Source: CAD feature listing. Evaluate the final solid. Frame: model axes, mm. A direction names the side the tool comes from. Give positions to 0.01 mm unless a question says otherwise; leave off trailing zeros. Loops run counter-clockwise (first coordinate to the right, second up) from the corner with the lowest first, then second, coordinate; pieces in that order, holes last. Notation, with made-up numbers: M -13.5,31.5 L -9.5,31.5 A19 cw -9.5,49.5 Z; hole C -38.5,30.25 d9. An arc over 180 degrees is marked long. Put each result on its own line as item: value. Start each with the question number.
```python
from build123d import *

# Parameters (mm, degrees)
EXTRUDE_1_DEPTH     = 28
SKETCH_2_R          = 11
EXTRUDE_2_DEPTH     = 2
SKETCH_3_R          = 2.5
EXTRUDE_3_DEPTH     = 13
SKETCH_4_R          = 1.3
CUT_EXTRUDE_1_DEPTH = 5


with BuildPart() as part:
    # 草图1 → 凸台-拉伸1 (new body)
    with BuildSketch(Plane(origin=(0, 0, 0), x_dir=(1, 0, 0), z_dir=(0, 1, 0))):
        with BuildLine():
            Line((-11.5, 14), (11.5, 14))
            ThreePointArc((11.5, 14), (13.267766953, 13.267766953), (14, 11.5))
            Line((14, 11.5), (14, -11.5))
            ThreePointArc((14, -11.5), (13.267766953, -13.267766953), (11.5, -14))
            Line((11.5, -14), (-11.5, -14))
            ThreePointArc((-11.5, -14), (-13.267766953, -13.267766953), (-14, -11.5))
            Line((-14, -11.5), (-14, 11.5))
            ThreePointArc((-14, 11.5), (-13.267766953, 13.267766953), (-11.5, 14))
        make_face()
    extrude(amount=EXTRUDE_1_DEPTH)

    # 草图2 → 凸台-拉伸2 (add)
    with BuildSketch(Plane(origin=(0, 28, 0), x_dir=(-1, 0, 0), z_dir=(0, 1, 0))):
        with Locations(Location((0, 0, 0), (0, 0, 90))):
            Circle(SKETCH_2_R)
    extrude(amount=EXTRUDE_2_DEPTH)

    # 草图3 → 凸台-拉伸3 (add)
    with BuildSketch(Plane(origin=(0, 30, 0), x_dir=(-1, 0, 0), z_dir=(0, 1, 0))):
        with Locations(Location((0, 0, 0), (0, 0, 270))):
            Circle(SKETCH_3_R)
    extrude(amount=EXTRUDE_3_DEPTH)

    # 草图4 → 切除-拉伸1 (cut)
    with BuildSketch(Plane(origin=(0, 28, 0), x_dir=(-1, 0, 0), z_dir=(0, 1, 0))):
        with Locations(Location((11.5, 11.5, 0), (0, 0, 90))):
            Circle(SKETCH_4_R)
        with Locations(Location((11.5, -11.5, 0), (0, 0, 90))):
            Circle(SKETCH_4_R)
        with Locations(Location((-11.5, -11.5, 0), (0, 0, 90))):
            Circle(SKETCH_4_R)
        with Locations(Location((-11.5, 11.5, 0), (0, 0, 90))):
            Circle(SKETCH_4_R)
    extrude(amount=-CUT_EXTRUDE_1_DEPTH, mode=Mode.SUBTRACT)


solid = part.part
```
1. Section D-D, the plane x = 3. Output: boundary loops of the cut face in (y, z).
2. Set-up query: faces 1 (the face through (14, 14, 0)), 2 (the face through (12.79, 25.54, -11.67)). Return all of +Z, -Z, +X, -X, +Y, -Y with unobstructed straight access to the full face (end or side cutting, diameter ignored); none if empty.
3. Section A-A, the plane x = 0. Output: boundary loops of the cut face in (y, z), plus the area to 3 significant figures.
4. Contact query for flat-ended pins moving along their axis: pin 1 (3 mm diameter, centred on x = 11, z = -11, fed in from +Y); pin 2 (2 mm diameter, centred on x = -1.5, y = 32.5, fed in from -Z); pin 3 (3 mm diameter, centred on x = -11.5, z = 11.5, fed in from -Y); pin 4 (2.5 mm diameter, centred on x = -11.5, z = -11.5, fed in from +Y). Output: stop coordinate, or through.
5. Ray query, line 1 (X direction, y = 26.25, z = 11.5); line 2 (Y direction, x = 9.75, z = -3.5); line 3 (Y direction, x = 5.25, z = 12.75). Return the intervals inside material, ascending.
6. Pull-direction query (X, two-part tool) for faces 3 (the face through (2.44, 36.41, 0.54)), 4 (the face through (-10.21, 25.54, -11.67)), 5 (the face through (0, 14, 14)); classes: released by +X, released by -X, zero draft, split by the parting line, or undercut.
7. Section B-B, the plane y = 26. Output: boundary loops of the cut face in (x, z), plus the area to 3 significant figures.
8. Section C-C, the plane z = 0. Output: boundary loops of the cut face in (x, y), plus the area to 3 significant figures.
Results found:
1. outline: M 0,-14 L 28,-14 L 28,-10.58 L 30,-10.58 L 30,10.58 L 28,10.58 L 28,14 L 0,14 Z
2. face 1: +Z, -Z, +X, +Y, -Y
2. face 2: +Y
3. outline: M 0,-14 L 28,-14 L 28,-11 L 30,-11 L 30,-2.5 L 43,-2.5 L 43,2.5 L 30,2.5 L 30,11 L 28,11 L 28,14 L 0,14 Z
3. area: 893 mm²
4. pin 1: y = 28
4. pin 2: z = -2.45
4. pin 3: y = 0
4. pin 4: y = 23
5. line 1: -14 to -12.8, -10.2 to 10.2, 12.8 to 14
5. line 2: 0 to 30
5. line 3: 0 to 28
6. face 3: split by the parting line
6. face 4: undercut
6. face 5: zero draft
7. outline: M -14,-11.5 A2.5 ccw -11.5,-14 L 11.5,-14 A2.5 ccw 14,-11.5 L 14,11.5 A2.5 ccw 11.5,14 L -11.5,14 A2.5 ccw -14,11.5 Z; hole C -11.5,-11.5 d2.6; hole C -11.5,11.5 d2.6; hole C 11.5,-11.5 d2.6; hole C 11.5,11.5 d2.6
7. area: 757 mm²
8. outline: M -14,0 L 14,0 L 14,28 L 11,28 L 11,30 L 2.5,30 L 2.5,43 L -2.5,43 L -2.5,30 L -11,30 L -11,28 L -14,28 Z
8. area: 893 mm²
